For this review, use the dimensioned drawing (mm, ordinates from the lowest corner) and the shaded views. Coordinates: 2 decimals unless noted, no trailing zeros. Loops run counter-clockwise (first coordinate to the right, second up) from the corner with the lowest first, then second, coordinate; pieces in that order, holes last. Notation, with made-up numbers: M 73,43.5 L 87,43.5 A17 ccw 87,63.5 Z; hole C 67,7 d11. An arc over 180 degrees is marked long. One line per item, written item: value.
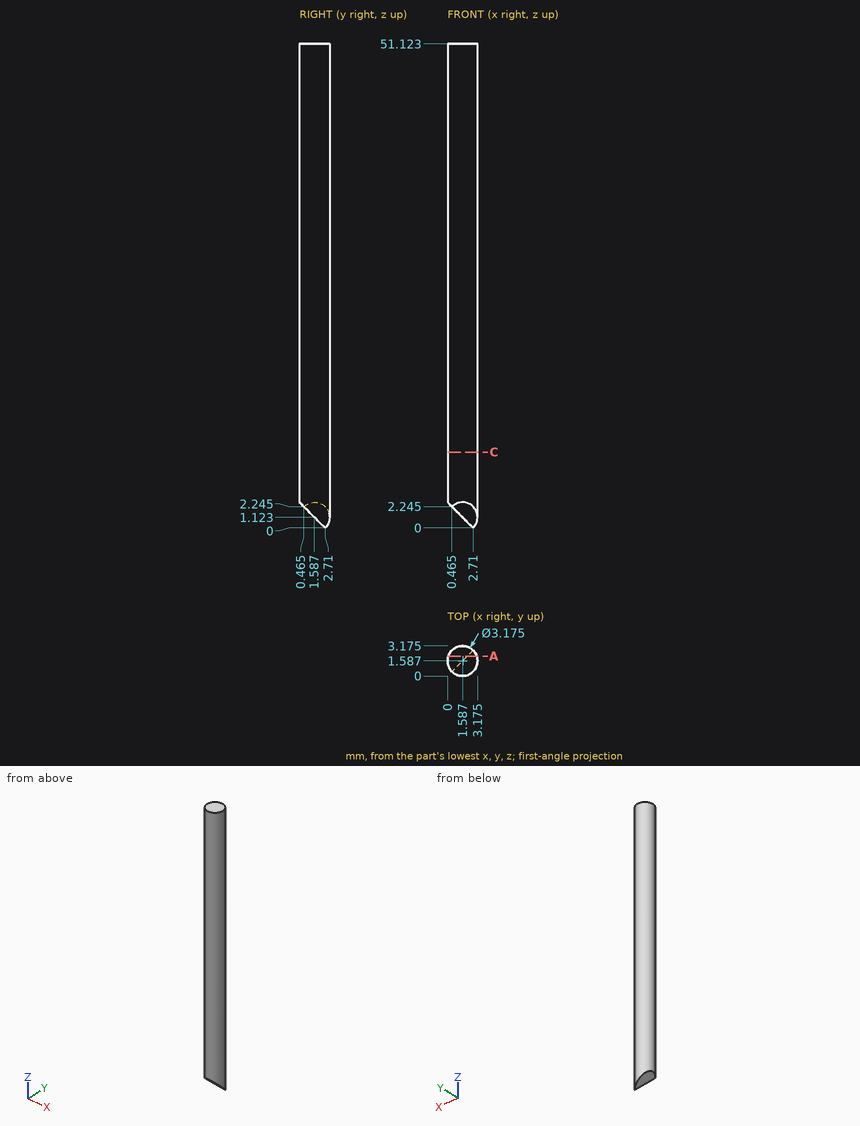
(1) Insertion check: pin 1 (1 mm diameter, centred on y = 0.5, z = 34.5, fed in from -X); pin 2 (1.5 mm diameter, centred on y = 2.5, z = 20, fed in from -X); pin 3 (1 mm diameter, centred on x = 2, z = 32.5, fed in from -Y). Each pin has a flat end and moves straight along its axis. Give the tip position at first contact, or say it passes through.
Reply:
pin 1: stops at x = 0.11
pin 2: stops at x = 0.01
pin 3: stops at y = 0
(2) We need section A-A on y = 2.1. State the section outline as (x, z) points (1 decimal), then the cut area to 3 significant figures.
Reply:
outline: M 0.1,2.6 L 2.1,0.6 L 3.1,0.6 L 3.1,51.1 L 0.1,51.1 Z
area: 150 mm2
(3) We need section C-C on z = 8. State the section outline as (x, y) points (1 decimal).
Reply:
outline: C 1.6,1.6 d3.2
(4) To check wall thickness, follow line 1 along Y through (x, z) = (1.75, 20.5); line 2 along X through (y, z) = (1.45, 40) (1 decimal); line 3 along Y through (x, z) = (2.6, 35) (1 decimal). State the ranges of each line that lie inside material, in increasing order. Write a range as [from, to].
Reply:
line 1: y = [0.01, 3.17]
line 2: x = [0, 3.2]
line 3: y = [0.4, 2.8]
